Model file for the job. Use its own axes, mm. A direction names the side the tool comes from. Round coordinates to 2 decimals unless told otherwise and drop trailing zeros. Loops run counter-clockwise (first coordinate to the right, second up) from the corner with the lowest first, then second, coordinate; pieces in that order, holes last. Notation, with made-up numbers: (52, 12.25) -> (62, 12.25) arc R35 cw to (62, 45.25) -> close; hole circle Ø10 at (-35, 50.5). An arc over 180 degrees is marked (long way). Use a Markdown table: item, result.
from build123d import *

# Parameters (mm, degrees)
SKETCH_1_R          = 3
SKETCH_1_R_2        = 2
EXTRUDE_1_DEPTH     = 5
SKETCH_2_R          = 0.5
CUT_EXTRUDE_1_DEPTH = 5
SKETCH_3_R          = 0.6
CUT_EXTRUDE_2_DEPTH = 2.5


with BuildPart() as part:
    # 草图1 → 凸台-拉伸1 (new body)
    with BuildSketch(Plane.XY):
        Circle(SKETCH_1_R)
        Circle(SKETCH_1_R_2, mode=Mode.SUBTRACT)
    extrude(amount=EXTRUDE_1_DEPTH)

    # 草图2 → 切除-拉伸1 (cut)
    with BuildSketch(Plane(origin=(0, 0, 0), x_dir=(1, 0, 0), z_dir=(0, 1, 0))):
        with Locations((0, -2.5)):
            Circle(SKETCH_2_R)
    extrude(amount=-CUT_EXTRUDE_1_DEPTH, mode=Mode.SUBTRACT)

    # 草图3 → 切除-拉伸2 (cut)
    with BuildSketch(Plane(origin=(0, 0, 0), x_dir=(1, 0, 0), z_dir=(0, 1, 0))):
        with Locations((0, -2.5)):
            Circle(SKETCH_3_R)
    extrude(amount=-CUT_EXTRUDE_2_DEPTH, mode=Mode.SUBTRACT)


solid = part.part
Q1. Drill centre lines: L1, parallel to Z at x = 0, y = -2.65; L2, parallel to Y at x = 0, z = 3.2; L3, parallel to Y at x = 0.5, z = 0.3. Where is each one in solid material? Low to high. Write a range as from..to.
Results list:
| item | result |
|---|---|
| L1 | z = 0..2, 3..5 |
| L2 | y = -3..-2, 2..3 |
| L3 | y = -2.96..-1.94, 1.94..2.96 |
Q2. Band-saw the part on A-A, the plane y = 0. Give the cut face in (x, z).
Results list:
| item | result |
|---|---|
| outline | (-3, 0) -> (-2, 0) -> (-2, 5) -> (-3, 5) -> close; (2, 0) -> (3, 0) -> (3, 5) -> (2, 5) -> close |
Q3. Band-saw the part on C-C, the plane z = 1.45. Give the cut face in (x, y).
Results list:
| item | result |
|---|---|
| outline | circle Ø6 at (0, 0); hole circle Ø4 at (0, 0) |
Q4. Flat gauge pins, fed straight in: pin 1 (1 mm diameter, centred on x = 2, z = 2, fed in from -Y); pin 2 (1.5 mm diameter, centred on x = -2, z = 4, fed in from -Y). Where does each tip first touch, or does it go through?
Results list:
| item | result |
|---|---|
| pin 1 | stops at y = -2.6 |
| pin 2 | stops at y = -2.73 |
Q5. Pull direction X, two halves, no side cores. Call faces 1 (the face through (-3, 0, 2)), 2 (the face through (1, -2, 0)), 3 (the face through (0.572, -2.2, 2.32)): released by +X, released by -X, zero draft, split by the parting line, or undercut.
Results list:
| item | result |
|---|---|
| face 1 | split by the parting line |
| face 2 | zero draft |
| face 3 | undercut |
Q6. Band-saw the part on B-B, the plane x = 0. Give the cut face in (y, z).
Results list:
| item | result |
|---|---|
| outline | (-3, 0) -> (-2, 0) -> (-2, 1.9) -> (-2.5, 1.9) -> (-2.5, 2) -> (-3, 2) -> close; (-3, 3) -> (-2.5, 3) -> (-2.5, 3.1) -> (-2, 3.1) -> (-2, 5) -> (-3, 5) -> close; (2, 0) -> (3, 0) -> (3, 5) -> (2, 5) -> close |
Q7. Tool access for faces 4 (the face through (-0.5, -2.7, 2.5)), 5 (the face through (1, -2, 5)): list every direction of +Z, -Z, +X, -X, +Y, -Y with a clear straight run to the whole face (end or side of a thin tool).
Results list:
| item | result |
|---|---|
| face 4 | -Y |
| face 5 | +Z, +X, -X, +Y, -Y |
Q8. Band-saw the part on D-D, the plane x = 1.25. Give the cut face in (y, z), plus the area to 3 significant figures.
Results list:
| item | result |
|---|---|
| outline | (-2.73, 0) -> (-1.56, 0) -> (-1.56, 5) -> (-2.73, 5) -> close; (1.56, 0) -> (2.73, 0) -> (2.73, 5) -> (1.56, 5) -> close |
| area | 11.7 mm² |
